Check sheet for the modelled part. Datum: model origin and axes. Units: mm. A direction names the side the tool comes from. Give positions to 0.01 mm unless a question says otherwise; leave off trailing zeros. Order: outer loops, then holes, each group sorted by start corner. A loop starts at its lowest first (then second) coordinate and runs counter-clockwise, first axis right, second up.
Item 1: Sectioned sample at B-B on x = -34.15. Record the boundary of the cut face in (y, z), and give its area (3 significant figures).
Item 2: Sectioned sample at A-A on y = 13. Record the boundary of the cut face in (x, z), and give its area (3 significant figures).
Item 3: Access from +Z, -Z, +X, -X, +Y, -Y to the whole of each face (thin tool, end or side, straight path). Record for faces 1 (the flat face through (34, 10, -14.96)), 2 (the flat face through (-42.5, 13, -17)), 3 (the flat face through (-34, 10, -14.96)).
Item 4: Sectioned sample at D-D on x = 0. Record the boundary of the cut face in (y, z), and give its area (3 significant figures).
Item 5: Release check for a two-part mould opening along X. For faces 4 (the cylindrical face through (36.9, 12.9, -16.2)), 5 (the flat face through (2.9, 26, -14.4)), 6 (the cylindrical face through (-19.775, 12.832, -8.663)) record: released by +X, released by -X, zero draft, split by the parting line, or undercut.
Item 6: Material ranges on line 1 along X through (y, z) = (13, -16.4); line 2 along Z through (x, y) = (0, 10.75); line 3 along Y through (x, z) = (-34.15, -16.3), recorded low to high.
Item 7: Gauge pin test, flat ends, axial feed: P1, Ø2, axis at y = 21.5, z = -10.5, coming from the -X side; P2, Ø8, axis at x = 32, y = 11.5, coming from the +Z side; P3, Ø5, axis at x = -34.15, y = 13, coming from the -Z side; P4, Ø2, axis at y = 5, z = 3, coming from the -X side. Record the tip position at first contact, or that the pin passes through.
Item 8: Sectioned sample at C-C on y = 20.75. Record the boundary of the cut face in (x, z).
Autodesk Fusion 360 part; units mm, degrees
sketch "Sketch1" plane through (0, 0, 0) normal (0, 1, 0) x (1, 0, 0)
  circle A0 centre (0, 0) radius 14.5
  circle A1 centre (0, 0) radius 17.5
  line L0 (0, 17.5) -> (28.7095, 17.5) construction
  line L1 (17.5, 0) -> (17.5, 17.5) construction
  line L2 (17.5, 0) -> (17.5, 17.5)
  line L3 (0, 17.5) -> (17.5, 17.5)
  line L4 (17.5, 17.5) -> (42.5, 17.5)
  line L5 (42.5, 17.5) -> (42.5, 14.96)
  line L6 (42.5, 14.96) -> (17.5, 14.96)
  line L7 (17.5, 14.96) -> (17.5, 17.5)
  line L8 (17.5, 14.96) -> (18.9859, 14.96) construction
  line L9 (17.5, 14.96) -> (25.8, 14.96) construction
  arc A2 (25.8, 14.96) -> (17.5, 0) centre (35.132, 0) ccw
  line L10 (0, -17.5) -> (0, 17.5) construction
  line L11 (17.5, 0) -> (-17.5, 0) construction
  arc A3 (-17.5, 0) -> (-25.8, 14.96) centre (-35.132, 0) ccw
  line L12 (-17.5, 0) -> (-17.5, 17.5)
  line L13 (-17.5, 14.96) -> (-25.8, 14.96) construction
  line L14 (-42.5, 14.96) -> (-17.5, 14.96)
  line L15 (-42.5, 17.5) -> (-42.5, 14.96)
  line L16 (-17.5, 17.5) -> (-42.5, 17.5)
  line L17 (0, 17.5) -> (-17.5, 17.5)
  dimension "d5" = 29
  dimension "d6" = 35
  dimension "d7" = 25
  dimension "d8" = 2.54
  dimension "d9" = 8.3
extrude "Extrude1" add sketch "Sketch1" along normal blind 26
sketch "Sketch3" plane through (0, 0, -14.96) normal (0, 0, 1) x (-1, 0, 0)
  line L0 (-25.8, 0) -> (-42.5, 0)
  line L1 (-42.5, 0) -> (-42.5, -26)
  line L2 (-42.5, -26) -> (-25.8, -26)
  line L3 (-25.8, -26) -> (-25.8, 0)
  line L4 (-25.8, -26) -> (-42.5, 0) construction
  line L5 (-42.5, -26) -> (-25.8, 0) construction
  circle A0 centre (-34.15, -13) radius 2.75
  dimension "d16" = 5.5
extrude "Extrude2" cut sketch "Sketch3" against normal up to surface (2.54 mm away) contours A0
mirror "Mirror1" about plane through (0, 0, 0) normal (1, 0, 0) of "Extrude2"
fillet "Fillet3" radius 1 13 edges at (-34.15, 0, -14.96) (-42.5, 13, -14.96) (-34.15, 26, -14.96) (-19.714, 0, -8.5541) (0, 0, 17.5) (19.714, 0, -8.5541) (-13.5187, 0, -5.2434) (34.15, 26, -14.96) (-19.714, 26, -8.5541) (0, 26, 17.5) (19.714, 26, -8.5541) (34.15, 0, -14.96) (42.5, 13, -14.96)
equation "InnerDiameter = 29 mm"
equation "OuterDiameter = 35 mm"
equation "Width = 26 mm"
equation "ScrewDiameter = 5.5 mm"
equation "d5 = InnerDiameter"
equation "d6 = OuterDiameter"
equation "d10 = Width"
equation "d16 = ScrewDiameter"
Report:
1. outline: (0, -17.5) - (10.25, -17.5) - (10.25, -14.96) - (1, -14.96) arc R1 ccw to (0, -15.96) - close; (15.75, -17.5) - (26, -17.5) - (26, -15.96) arc R1 ccw to (25, -14.96) - (15.75, -14.96) - close
1. area: 51.6 mm2
2. outline: (-42.5, -17.5) - (-36.9, -17.5) - (-36.9, -14.96) - (-41.5, -14.96) arc R1 ccw to (-42.5, -15.96) - close; (-31.4, -17.5) - (31.4, -17.5) - (31.4, -14.96) - (25.8, -14.96) arc R17.63 cw to (17.5, 0) arc R17.5 ccw to (-17.5, 0) arc R17.63 cw to (-25.8, -14.96) - (-31.4, -14.96) - close; (36.9, -17.5) - (42.5, -17.5) - (42.5, -15.96) arc R1 ccw to (41.5, -14.96) - (36.9, -14.96) - close; hole circle Ø29 at (0, 0)
2. area: 605 mm2
3. face 1: +Z, +X, +Y, -Y
3. face 2: +Z, -Z, -X, +Y, -Y
3. face 3: +Z, -X, +Y, -Y
4. outline: (0, -17.5) - (26, -17.5) - (26, -14.5) - (1, -14.5) arc R1 ccw to (0, -15.5) - close; (0, 15.5) arc R1 ccw to (1, 14.5) - (26, 14.5) - (26, 16.5) arc R1 ccw to (25, 17.5) - (1, 17.5) arc R1 ccw to (0, 16.5) - close
4. area: 155 mm2
5. face 4: undercut
5. face 5: zero draft
5. face 6: released by -X
6. line 1: x = -42.5 to -36.9, -31.4 to 31.4, 36.9 to 42.5
6. line 2: z = -17.5 to -14.5, 14.5 to 17.5
6. line 3: y = 0 to 10.25, 15.75 to 26
7. P1: stops at x = -21.77
7. P2: stops at z = -14.96
7. P3: passes through
7. P4: stops at x = -17.39
8. outline: (-42.5, -17.5) - (42.5, -17.5) - (42.5, -15.96) arc R1 ccw to (41.5, -14.96) - (25.8, -14.96) arc R17.63 cw to (17.5, 0) arc R17.5 ccw to (-17.5, 0) arc R17.63 cw to (-25.8, -14.96) - (-41.5, -14.96) arc R1 ccw to (-42.5, -15.96) - close; hole circle Ø29 at (0, 0)
